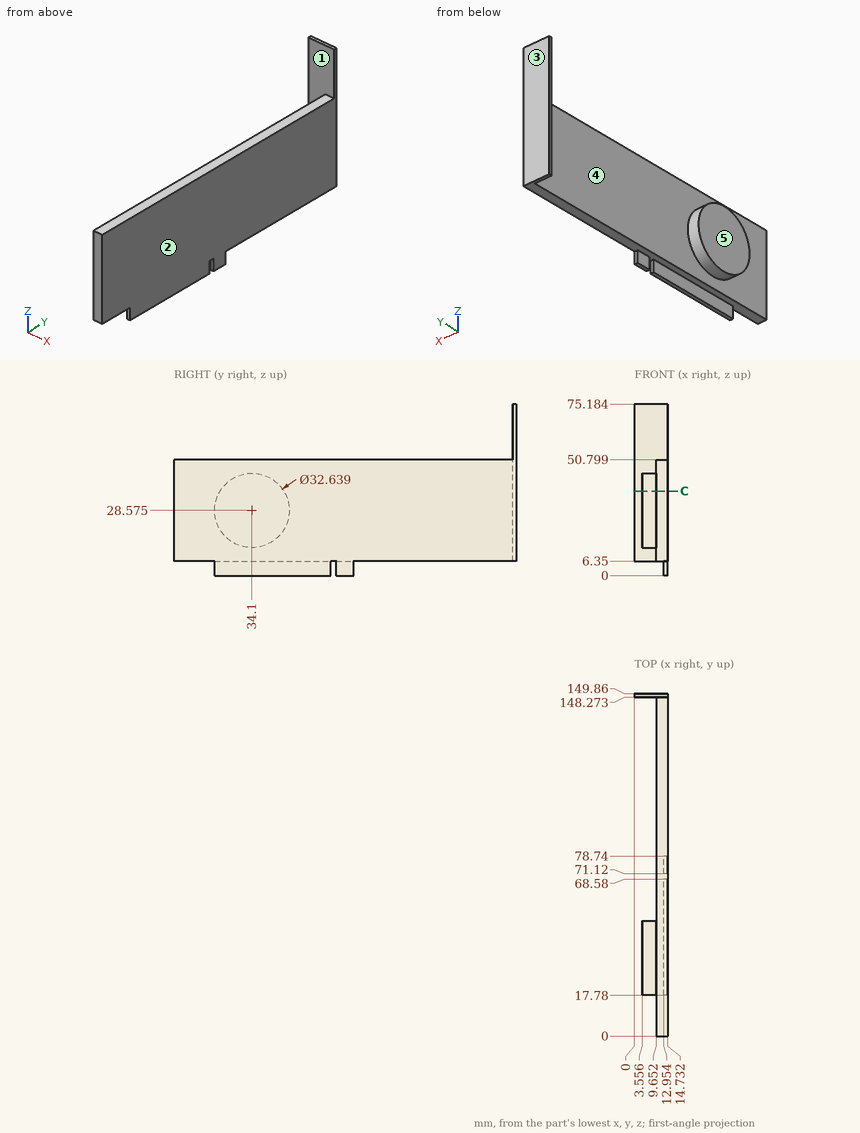
Answer from the drawing. Dimensions are ordinates in mm from the lowest x, y and z of the part. A direction names the side the tool comes from. Give positions to 0.01 mm unless a question says otherwise; leave off trailing zeros. Loops run counter-clockwise (first coordinate to the right, second up) from the corner with the lowest first, then second, coordinate; pieces in that order, holes last.
Item 1: Each of these flat-tipped pins is pushed along its axis until it touches: pin 1 Ø3 at (y, z) = (40.5, 39.5) entering from -X; pin 2 Ø1.4 at (x, z) = (14, 4.5) entering from +Y; pin 3 Ø4 at (x, y) = (13, 57.5) entering from +Z. Where does it stop, or does it pass through?
Derived:
pin 1: stops at x = 3.56
pin 2: stops at y = 78.74
pin 3: stops at z = 50.8
Item 2: Determine the mould class of the marked faces 3, 4 and 5 for opening direction Y: +Y half, -Y half, draft (parallel to the pull), parting line (faces both ways), or undercut.
Derived:
face 3: +Y half
face 4: undercut
face 5: draft
Item 3: A cutting plane is placed at C-C (z = 37). Give the vertices of the cut face in (x, y) (1 decimal), then the cut area to 3 significant figures.
Derived:
outline: (0, 148.3) - (9.7, 148.3) - (9.7, 48.1) - (3.6, 48.1) - (3.6, 20.1) - (9.7, 20.1) - (9.7, 0) - (14.7, 0) - (14.7, 149.9) - (0, 149.9) - close
area: 947 mm2
Item 4: A tool of negligible diameter and unlimited length cuts with its end or side. For the marked faces 1 and 2, from which of +Z, -Z, +X, -X, +Y, -Y can it reach the whole face along a straight path? Write none if from no direction.
Derived:
face 1: +Z, -X
face 2: +Z, -Z, +X, +Y, -Y
Item 5: Find the intervals of material crossed by line 1 along X through (y, z) = (105, 28); line 2 along Z through (x, y) = (13.75, 14); line 3 along Y through (x, z) = (7, 26) (1 decimal), in increasing order.
Derived:
line 1: x = 9.65 to 14.73
line 2: z = 6.35 to 50.8
line 3: y = 18 to 50.2, 148.3 to 149.9
